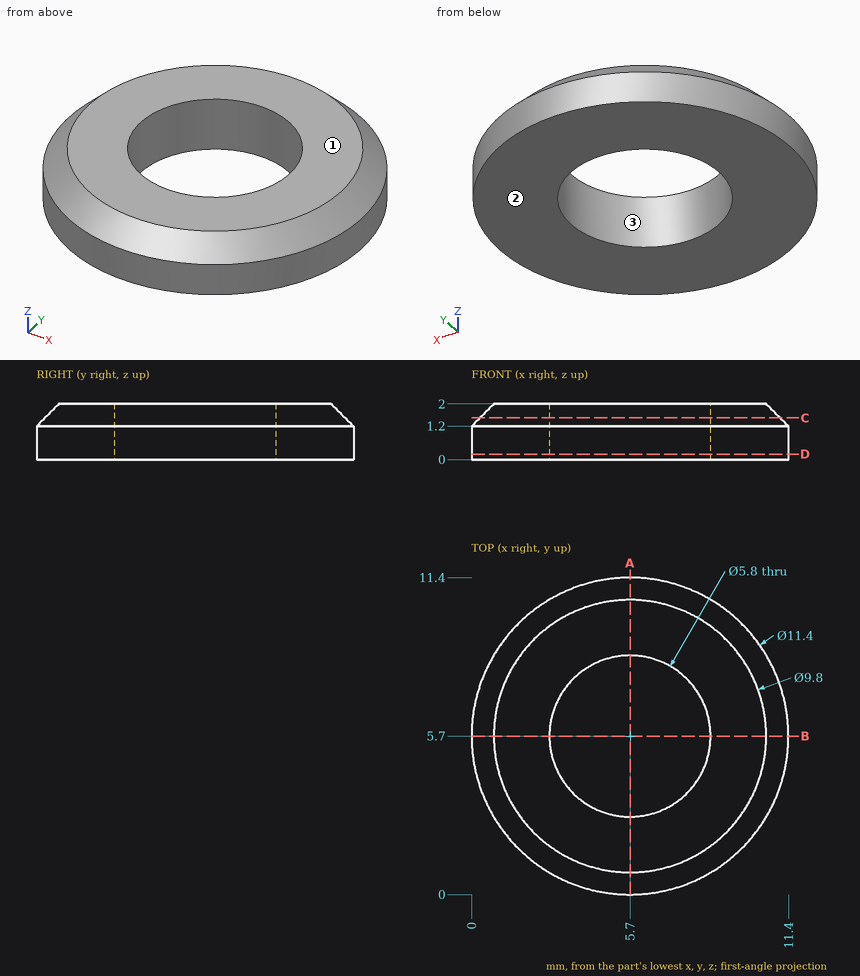
Source: three-view drawing plus pictorial views. Frame: mm from the lowest corner of the part. Round coordinates to 2 decimals unless told otherwise and drop trailing zeros. Loops run counter-clockwise (first coordinate to the right, second up) from the corner with the lowest first, then second, coordinate; pieces in that order, holes last. Notation, with made-up numbers: M 49.25,-21 L 60.25,-21 A24 ccw 60.25,11 Z; hole C 58,-35.75 d7. An arc over 180 degrees is marked long. Put each result on its own line as item: value. Start each with the question number.
(1) Section query D-D (z = 0.2). Return loops of the section in (x, y).
(2) Draft query along Z for the marked faces 1, 2 and 3. Return one class per face: +Z half, -Z half, draft (parallel to the pull), parting line (faces both ways), or undercut.
(3) Material intervals for line 1 along Y through (x, z) = (5.7, 0.95); line 2 along Y through (x, z) = (5.7, 1.65); line 3 along X through (y, z) = (5.5, 0.8), sorted ascending. Write a range as [from, to].
(4) Contact query for flat-ended pins moving along their axis: pin 1 Ø3.5 at (x, y) = (5.7, 5.7) entering from -Z; pin 2 Ø1 at (y, z) = (2, 1) entering from -X. Output: stop coordinate, or through.
(5) Section query A-A (x = 5.7). Return loops of the section in (y, z).
(6) Section query C-C (z = 1.5). Return loops of the section in (x, y), then the cut area to 3 significant figures.
Findings below:
1. outline: C 5.7,5.7 d11.4; hole C 5.7,5.7 d5.8
2. face 1: +Z half
2. face 2: -Z half
2. face 3: draft
3. line 1: y = [0, 2.8], [8.6, 11.4]
3. line 2: y = [0.45, 2.8], [8.6, 10.95]
3. line 3: x = [0, 2.81], [8.59, 11.4]
4. pin 1: passes through
4. pin 2: stops at x = 0.98
5. outline: M 0,0 L 2.8,0 L 2.8,2 L 0.8,2 L 0,1.2 Z; M 8.6,0 L 11.4,0 L 11.4,1.2 L 10.6,2 L 8.6,2 Z
6. outline: C 5.7,5.7 d10.8; hole C 5.7,5.7 d5.8
6. area: 65.2 mm2
